Verification items for the finished model (mm, model axes). A direction names the side the tool comes from. Coordinates: 2 decimals unless noted, no trailing zeros. Loops run counter-clockwise (first coordinate to the right, second up) from the corner with the lowest first, then second, coordinate; pieces in that order, holes last. Notation, with made-up numbers: (-12.75, 3) -> (27.25, 3) arc R16 ccw to (27.25, 11) -> close; hole circle Ø2 at (19.25, 1.25). An arc over 180 degrees is marked (long way). Answer as a JSON object with one key per item and string values. Group by question number.
Q1. Scan lines: L1, parallel to Y at x = 0, z = -0.3; L2, parallel to Z at x = 4.5, y = -3; L3, parallel to Z at x = 1, y = 3.5 (3 decimals). Record each from-to range of solid material in increasing order.
Q2. Release check for a two-part mould opening along X. For faces 3 (the flat face through (2, -2, -2)), 4 (the cylindrical face through (-5.794, 0.255, 1.606)), 5 (the cylindrical face through (-0.54, 2.44, -0.03)) record: released by +X, released by -X, zero draft, split by the parting line, or undercut.
Q3. Cross-section at C-C on z = -1.25. Record the boundary of the cut face in (x, y).
Q4. Set-up check for faces 1 (the cylindrical face through (-1.08, 4.88, -0.42)), 2 (the flat face through (-2, -4, -2)): record each of +Z, -Z, +X, -X, +Y, -Y from which the full face is reachable in a straight line by a thin tool's end or side.
Q5. Gauge pin test, flat ends, axial feed: pin 1 Ø1 at (x, z) = (1, -1) entering from +Y; pin 2 Ø2.5 at (x, y) = (2, -1) entering from +Z. Record the tip position at first contact, or that the pin passes through.
Q6. Cross-section at A-A on x = 0. Record the boundary of the cut face in (y, z) (3 decimals), and give its area (3 significant figures).
Q7. Cross-section at D-D on y = 3. Record the boundary of the cut face in (x, z) (3 decimals), and give its area (3 significant figures).
Autodesk Inventor part; units mm, degrees
ref_plane "YZ Plane" through (0, 0, 0) normal (1, 0, 0) x (0, 1, 0)
ref_plane "XZ Plane" through (0, 0, 0) normal (0, 1, 0) x (-1, 0, 0)
ref_plane "XY Plane" through (0, 0, 0) normal (0, 0, 1) x (1, 0, 0)
sketch "Sketch1" plane through (0, 0, 0) normal (0, 0, 1) x (1, 0, 0)
  circle A0 centre (0, 0) radius 2.5
  circle A1 centre (0, 0) radius 5
  circle A2 centre (0, 0) radius 4.25
  circle A3 centre (0, 0) radius 3.25
  dimension "d0" = 5
  dimension "d1" = 10
  dimension "d2" = 0.75
  dimension "d3" = 0.75
extrude "Extrusion1" add sketch "Sketch1" along normal mid plane 4
extrude "Extrusion2" add sketch "Sketch1" along normal mid plane 3.75 contours A2
sketch "Sketch2" plane through (0, 0, 2) normal (0, 0, 1) x (1, 0, 0)
  circle A0 centre (0, 0) radius 5
  circle A1 centre (0, 0) radius 5.8
  dimension "d8" = 11.6
extrude "Extrusion3" add sketch "Sketch2" against normal blind 0.8
properties part number "MF105ZZ" material "Steel, Carbon"
Computed values:
{
 "1": {"L1": "y = -5 to -2.5, 2.5 to 5", "L2": "z = 1.2 to 2", "L3": "z = -1.875 to 1.875"},
 "2": {"face 3": "zero draft", "face 4": "split by the parting line", "face 5": "undercut"},
 "3": {"outline": "circle Ø10 at (0, 0); hole circle Ø5 at (0, 0)"},
 "4": {"face 1": "-Z", "face 2": "-Z, +X, -X, +Y, -Y"},
 "5": {"pin 1": "stops at y = 4.97", "pin 2": "stops at z = 2"},
 "6": {"outline": "(-5.8, 1.2) -> (-5, 1.2) -> (-5, -2) -> (-4.25, -2) -> (-4.25, -1.875) -> (-3.25, -1.875) -> (-3.25, -2) -> (-2.5, -2) -> (-2.5, 2) -> (-3.25, 2) -> (-3.25, 1.875) -> (-4.25, 1.875) -> (-4.25, 2) -> (-5.8, 2) -> close; (2.5, -2) -> (3.25, -2) -> (3.25, -1.875) -> (4.25, -1.875) -> (4.25, -2) -> (5, -2) -> (5, 1.2) -> (5.8, 1.2) -> (5.8, 2) -> (4.25, 2) -> (4.25, 1.875) -> (3.25, 1.875) -> (3.25, 2) -> (2.5, 2) -> close", "area": "20.8 mm²"},
 "7": {"outline": "(-4.964, 1.2) -> (-4, 1.2) -> (-4, -2) -> (-3.01, -2) -> (-3.01, -1.875) -> (-1.25, -1.875) -> (-1.25, -2) -> (1.25, -2) -> (1.25, -1.875) -> (3.01, -1.875) -> (3.01, -2) -> (4, -2) -> (4, 1.2) -> (4.964, 1.2) -> (4.964, 2) -> (3.01, 2) -> (3.01, 1.875) -> (1.25, 1.875) -> (1.25, 2) -> (-1.25, 2) -> (-1.25, 1.875) -> (-3.01, 1.875) -> (-3.01, 2) -> (-4.964, 2) -> close", "area": "32.7 mm²"}
}
